```python
from build123d import *

# Parameters (mm, degrees)
F0_R      = 28.575
F1_DEPTH  = 64
F2_DEPTH  = 44
F3_W      = 103.150376
F3_H      = 49.648258
F3_H_2    = 43.694865
F4_DEPTH  = 10
F5_W      = 114
F5_H      = 50
F6_DEPTH  = 22
F8_DEPTH  = 95.001
F9_R      = 11.1
F10_DEPTH = 22.001


with BuildPart() as f1:
    # F0 (on Top) → F1 (new body)
    with BuildSketch(Plane.XY):
        with BuildLine():
            Line((0.432614, 0), (0, 0))
            Line((0, 0), (0, 82))
            Line((0, 82), (0.432614, 82))
            ThreePointArc((0.432614, 82), (-88.709953, 41), (0.432614, 0))
        make_face()
        with Locations((-34.709953, 41)):
            Circle(F0_R, mode=Mode.SUBTRACT)
        with BuildLine():
            Line((0, 82), (0, 0))
            Line((0, 0), (0.432614, 0))
            ThreePointArc((0.432614, 0), (14.349698, 18.435632), (19.290047, 41))
            ThreePointArc((19.290047, 41), (14.349698, 63.564368), (0.432614, 82))
            Line((0.432614, 82), (0, 82))
        make_face()
    extrude(amount=F1_DEPTH)

    # F0 (on Top) → F2 (join)
    with BuildSketch(Plane.XY):
        with BuildLine():
            ThreePointArc((19.290047, 41), (14.349698, 18.435632), (0.432614, 0))
            Line((0.432614, 0), (139.29, 0))
            Line((139.29, 0), (139.29, 82))
            Line((139.29, 82), (0.432614, 82))
            ThreePointArc((0.432614, 82), (14.349698, 63.564368), (19.290047, 41))
        make_face()
    extrude(amount=F2_DEPTH)

    # F3 (on face) → F4 (cut)
    with BuildSketch(Plane.XY.offset(64)):
        with Locations((-34.709953, 0.175871)):
            Rectangle(F3_W, F3_H)
        with Locations((-34.709953, 78.847432)):
            Rectangle(F3_W, F3_H_2)
    extrude(amount=-F4_DEPTH, mode=Mode.SUBTRACT)

    # F5 (on face) → F6 (cut)
    with BuildSketch(Plane.XY.offset(44)):
        with Locations((82.29, 41)):
            Rectangle(F5_W, F5_H)
    extrude(amount=-F6_DEPTH, mode=Mode.SUBTRACT)

    # F7 (on face) → F8 (cut, through all)
    with BuildSketch(Plane.XZ):
        Polygon((139.29, 22), (139.29, 44), (127.29, 44), align=None)
    extrude(amount=-F8_DEPTH, mode=Mode.SUBTRACT)

    # F9 (on face) → F10 (cut, through all)
    with BuildSketch(Plane.XY.offset(22)):
        with Locations((54.29, 40.001135)):
            Circle(F9_R)
        with Locations((104.29, 40.001135)):
            Circle(F9_R)
    extrude(amount=-F10_DEPTH, mode=Mode.SUBTRACT)


solid = f1.part
```
Here's how the part is built. I have some questions about the finished solid (model axes, mm). A direction names the side the tool comes from. Coordinates: 2 decimals unless noted, no trailing zeros. Order: outer loops, then holes, each group sorted by start corner. A loop starts at its lowest first (then second) coordinate and runs counter-clockwise, first axis right, second up. Notation, with made-up numbers: (77.25, -30.75) - (123.25, -30.75) arc R25 ccw to (123.25, -12.75) - close; hole circle Ø7 at (38.25, 59). An arc over 180 degrees is marked (long way). One line per question, with ' | ' between items. Start each with the question number.
1. If we section it at A-A (x = 71): Write out the boundary of the cut face in (y, z), and give its area (3 significant figures).
2. Which directions (+Z, -Z, +X, -X, +Y, -Y) give clear straight access to the entire face, cutting with the end or side of a thin tool? Please do faces 1 (the flat face through (3, 57, 59)), 2 (the flat face through (71, 82, 22)), 3 (the flat face through (-73, 25, 59)).
3. If we section it at C-C (z = 36): Write out the boundary of the cut face in (x, y) (3 decimals), and give its area (3 significant figures).
4. If we section it at B-B (y = 60): Write out the boundary of the cut face in (x, z), and give its area (3 significant figures).
5. If we mould it in two halves opening along X, with no side actions, what happens to faces 4 (the cylindrical face through (-8.31, 30.06, 31.55)), 5 (the flat face through (4, 41, 64)), 6 (the flat face through (139.29, 40, 11))? For each: released by +X, released by -X, zero draft, split by the parting line, or undercut.
6. I'm going to push flat-ended pins straight in: pin 1 Ø5 at (x, z) = (-76.5, 57) entering from -Y; pin 2 Ø1.5 at (x, z) = (79, 18.5) entering from +Y; pin 3 Ø11 at (y, z) = (39, 36.5) entering from +X. Where does each tip first touch, or does it pass through?
7. If we section it at D-D (x = -13.5): Write out the boundary of the cut face in (y, z).
8. Please list where these lines run through material, in increasing order: line 1 along Y through (x, z) = (65, 23.5); line 2 along Y through (x, z) = (104.29, 12); line 3 along Y through (x, z) = (21, 4.5). Write a range as [from, to].
Model answer:
1) outline: (0, 0) - (82, 0) - (82, 44) - (66, 44) - (66, 22) - (16, 22) - (16, 44) - (0, 44) - close | area: 2,510 mm²
2) face 1: +Z, +X, -X, +Y | face 2: +Z, -Z, +X, +Y | face 3: +Z, +X, -X, -Y
3) outline: (0.433, 0) - (131.654, 0) - (131.654, 16) - (25.29, 16) - (25.29, 66) - (131.654, 66) - (131.654, 82) - (0.433, 82) arc R54 ccw (long way) to start; hole circle Ø57.15 at (-34.71, 41) | area: 11,000 mm²
4) outline: (-85.26, 0) - (-56.05, 0) - (-56.05, 54) - (-85.26, 54) - close; (-13.37, 0) - (139.29, 0) - (139.29, 22) - (25.29, 22) - (25.29, 44) - (15.84, 44) - (15.84, 54) - (-13.37, 54) - close | area: 6,080 mm²
5) face 4: undercut | face 5: zero draft | face 6: released by +X
6) pin 1: stops at y = 25 | pin 2: stops at y = 82 | pin 3: stops at x = 25.29
7) outline: (-8.66, 0) - (21.85, 0) - (21.85, 54) - (-8.66, 54) - close; (60.15, 0) - (90.66, 0) - (90.66, 54) - (60.15, 54) - close
8) line 1: y = [0, 16], [66, 82] | line 2: y = [0, 28.9], [51.1, 82] | line 3: y = [0, 82]
